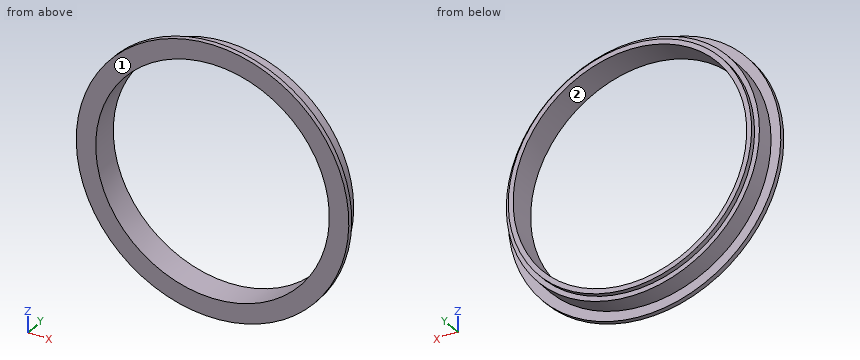
```python
from build123d import *

# Parameters (mm, degrees)
ESQUISSE1_R             = 28
BOSS_EXTRU_2_DEPTH      = 1
ESQUISSE2_R             = 26
ESQUISSE2_R_2           = 24
BOSS_EXTRU_5_DEPTH      = 4
ESQUISSE6_R             = 25
BOSS_EXTRU_6_DEPTH      = 1
ESQUISSE7_R             = 24
ENL_V_MAT_EXTRU_2_DEPTH = 41.049968789


with BuildPart() as part:
    # Esquisse1 → Boss.-Extru.2 (new body)
    with BuildSketch(Plane(origin=(0, 0, 0), x_dir=(1, 0, 0), z_dir=(0, 1, 0))):
        with Locations(Location((0, 0, 0), (0, 0, 270))):
            Circle(ESQUISSE1_R)
    extrude(amount=BOSS_EXTRU_2_DEPTH)

    # Esquisse2 → Boss.-Extru.5 (add)
    with BuildSketch(Plane(origin=(0, 1, 0), x_dir=(1, 0, 0), z_dir=(0, 1, 0))):
        with Locations(Location((0, 0, 0), (0, 0, 270))):
            Circle(ESQUISSE2_R)
        with Locations(Location((0, 0, 0), (0, 0, 270))):
            Circle(ESQUISSE2_R_2, mode=Mode.SUBTRACT)
    extrude(amount=BOSS_EXTRU_5_DEPTH)

    # Esquisse6 → Boss.-Extru.6 (add)
    with BuildSketch(Plane(origin=(0, 5, 0), x_dir=(1, 0, 0), z_dir=(0, 1, 0))):
        with Locations(Location((0, 0, 0), (0, 0, 270))):
            Circle(ESQUISSE6_R)
    extrude(amount=BOSS_EXTRU_6_DEPTH)

    # Esquisse7 → Enlèv. mat.-Extru.2 (cut, through all)
    with BuildSketch(Plane(origin=(0, 6, 0), x_dir=(1, 0, 0), z_dir=(0, 1, 0))):
        with Locations(Location((0, 0, 0), (0, 0, 270))):
            Circle(ESQUISSE7_R)
    extrude(amount=-ENL_V_MAT_EXTRU_2_DEPTH, mode=Mode.SUBTRACT)


solid = part.part
```
Can you work these out from the model? Positions are in its coordinate system, mm. Face numbers are marked on the shaded views. Round coordinates to 2 decimals unless told otherwise and drop trailing zeros. Loops run counter-clockwise (first coordinate to the right, second up) from the corner with the lowest first, then second, coordinate; pieces in that order, holes last. Notation, with made-up numbers: (-15, 48) -> (27, 48) arc R20 ccw to (27, 82) -> close; hole circle Ø6 at (20, 2). An arc over 180 degrees is marked (long way). One line per item, written item: value. Start each with the question number.
1. If we mould it in two halves opening along Z, with no side actions, what happens to the marked faces 1 and 2? For each: pulls with the +Z half, pulls with the -Z half, needs draft (parallel to the pull), parting line crosses it, or undercut.
2. If we section it at C-C, the plane y = 2.15: Write out the boundary of the cut face in (x, z).
3. If we section it at A-A, the plane z = 0: Write out the boundary of the cut face in (x, y).
4. For pin 1 (1 mm diameter, centred on x = 8, y = 4.5, fed in from -Z), with a flat end and sliding along its axis, tell me the tip position at first contact or that it passes through.
5. If we section it at B-B, the plane x = 0: Write out the boundary of the cut face in (y, z), then the cut area to 3 significant figures.
6. If I drill on probe 1 along Z at (x, y) = (-0.5, 1.4); probe 2 along X at (y, z) = (2, 0); probe 3 along Z at (x, y) = (7, 5.7), over which ranges is the centre line in solid material (lowest first)?
Calculated:
1. face 1: needs draft
1. face 2: undercut
2. outline: circle Ø52 at (0, 0); hole circle Ø48 at (0, 0)
3. outline: (-28, 0) -> (-24, 0) -> (-24, 6) -> (-25, 6) -> (-25, 5) -> (-26, 5) -> (-26, 1) -> (-28, 1) -> close; (24, 0) -> (28, 0) -> (28, 1) -> (26, 1) -> (26, 5) -> (25, 5) -> (25, 6) -> (24, 6) -> close
4. pin 1: stops at z = -24.89
5. outline: (0, -28) -> (1, -28) -> (1, -26) -> (5, -26) -> (5, -25) -> (6, -25) -> (6, -24) -> (0, -24) -> close; (0, 24) -> (6, 24) -> (6, 25) -> (5, 25) -> (5, 26) -> (1, 26) -> (1, 28) -> (0, 28) -> close
5. area: 26.0 mm²
6. probe 1: z = -26 to -23.99, 23.99 to 26
6. probe 2: x = -26 to -24, 24 to 26
6. probe 3: z = -24 to -22.96, 22.96 to 24
